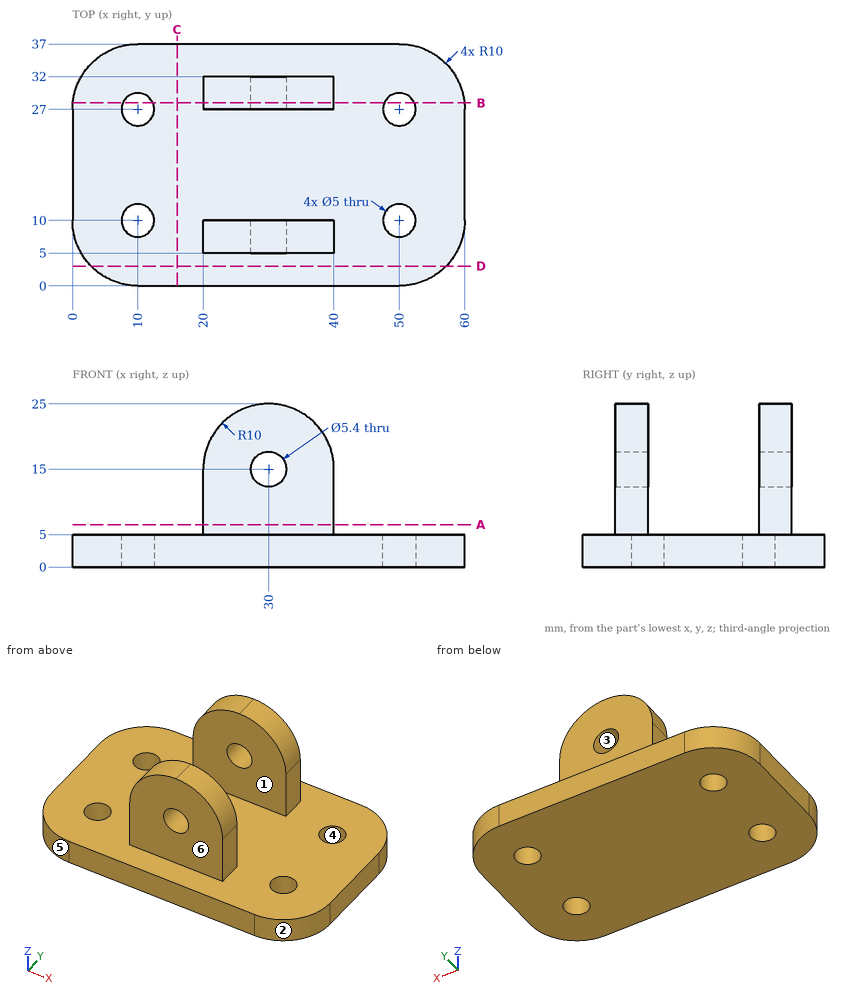
Input: dimensioned drawing with shaded views. Units: mm. Origin: part minimum x, y, z. A direction names the side the tool comes from. Give positions to 0.01 mm unless a question says otherwise; leave off trailing zeros. Write each loop counter-clockwise with the first axis right and the second up, starting at its lowest first coordinate (ties: lowest second). Pieces come first, ordered by that corner, then holes.
1. Line query: probe 1 along Y at (x, z) = (50, 1.2); probe 2 along X at (y, z) = (28.5, 15); probe 3 along Y at (x, z) = (28, 21). Output: solid intervals per line, ascending.
2. Section query A-A, the plane z = 6.5. Return loops of the section in (x, y), then the cut area to 3 significant figures.
3. Section query D-D, the plane y = 3. Return loops of the section in (x, z), then the cut area to 3 significant figures.
4. Reachability of the marked faces 5 and 6 from +Z, -Z, +X, -X, +Y, -Y: full face, straight path, thin tool, end or side. Return the list, or none.
5. Draft query along Y for the marked faces 1, 2, 3 and 4. Return one class per face: released by +Y, released by -Y, zero draft, split by the parting line, or undercut.
6. Section query C-C, the plane x = 16. Return loops of the section in (y, z).
7. Section query B-B, the plane y = 28. Count the separate pieces of the cut face and the enclosed holes in it, then the cut area to 3 significant figures.
8. Pin query (flat end, axial travel): P1, Ø11, axis at x = 18, y = 12.5, coming from the +Z side; P2, Ø1.5, axis at y = 28.5, z = 8.5, coming from the +X side; P3, Ø10, axis at x = 31.5, z = 11, coming from the +Y side; P4, Ø10, axis at x = 43, y = 18.5, coming from the -Z side. Return the tip coordinate at first contact, or that it passes through.
Computed:
1. probe 1: y = 0 to 7.5, 12.5 to 24.5, 29.5 to 37
1. probe 2: x = 20 to 27.3, 32.7 to 40
1. probe 3: y = 5 to 10, 27 to 32
2. outline: (20, 5) - (40, 5) - (40, 10) - (20, 10) - close; (20, 27) - (40, 27) - (40, 32) - (20, 32) - close
2. area: 200 mm2
3. outline: (2.86, 0) - (57.14, 0) - (57.14, 5) - (2.86, 5) - close
3. area: 271 mm2
4. face 5: +Z, -Z, -X, -Y
4. face 6: +Z, +X, -X, -Y
5. face 1: undercut
5. face 2: released by -Y
5. face 3: zero draft
5. face 4: undercut
6. outline: (0, 0) - (37, 0) - (37, 5) - (0, 5) - close
7. separate pieces: 3
7. enclosed holes: 1
7. area: 588 mm2
8. P1: stops at z = 22.04
8. P2: stops at x = 40
8. P3: stops at y = 32
8. P4: stops at z = 0
